For this review, take the finished solid that the model builds, in its own axes (mm). A direction names the side the tool comes from. Give positions to 0.01 mm unless a question says otherwise; leave off trailing zeros. Write each loop counter-clockwise with the first axis right and the second up, starting at its lowest first coordinate (ties: lowest second). Pieces come first, ordered by that corner, then holes. Notation, with made-up numbers: M 7.5,89.5 L 59.5,89.5 A14 cw 59.5,116.5 Z; hole C 72,-34 d1. An arc over 180 degrees is marked long. One line per item, written item: value. Start each with the question number.
Item 1: Consider section C-C, the plane y = -7.5. Write out the cut boundary in (x, z), and give its area (3 significant figures).
Item 2: Consider section A-A, the plane z = 0. Write out the cut boundary in (x, y).
Item 3: Consider section B-B, the plane x = 0. Write out the cut boundary in (y, z).
Item 4: Mouldability with a two-part tool opening along Y and no side actions: class faces 1 (the face through (4, 0, 7)), 2 (the face through (4, -20, 7)), 3 (the face through (-6.347, -5.746, 5.319)) as released by +Y, released by -Y, zero draft, split by the parting line, or undercut.
Item 5: Clearance check with flat-ended pins moving along their axes: pin 1 Ø1 at (y, z) = (-3, 6.5) entering from -X; pin 2 Ø6 at (x, y) = (0, -7.5) entering from +Z; pin 3 Ø4 at (y, z) = (-3.5, 7) entering from -X; pin 4 Ø2 at (y, z) = (-4.5, -5.5) entering from +X. State where each tip first meets the part, or that it passes through.
Item 6: To check wall thickness, follow probe 1 along Y at (x, z) = (0, 8.1); probe 2 along X at (y, z) = (-3.5, 0.25). State the ranges of each line that lie inside material, in increasing order.
Item 7: Tool access review of faces 4 (the face through (-1.8, -6.9, 8.2)), 5 (the face through (4.153, -9.86, -7.985)): name each direction out of +Z, -Z, +X, -X, +Y, -Y from which nothing blocks a thin tool from reaching the whole face with its end or side.
Item 8: Consider section D-D, the plane y = -12.5. Write out the cut boundary in (x, z), and give its area (3 significant figures).
```python
from build123d import *

# Parameters (mm, degrees)
F0_R     = 9
F0_R_2   = 7.75
F1_DEPTH = 20
F4_D     = 3.7973
F4_DEPTH = 3.021
F4_START = 0.20255
F4_TIP   = 1.1408240143
F8_D     = 3.7973
F8_DEPTH = 2
F8_START = 0.20255
F8_TIP   = 1.1408240143


with BuildPart() as f1:
    # F0 (on Front) → F1 (new body)
    with BuildSketch(Plane.XZ):
        Circle(F0_R)
        Circle(F0_R_2, mode=Mode.SUBTRACT)
    extrude(amount=F1_DEPTH)

    # F4
    # its depths count from where the whole tool has entered the part; down to there all is cleared
    with Locations(Plane.XY.offset(9).offset(-F4_START)):
        with Locations((0, -7.5)):
            Hole(F4_D / 2, depth=F4_DEPTH)
            with Locations((0, 0, -(F4_DEPTH + F4_TIP / 2))):  # 118° drill point
                Cone(0, F4_D / 2, F4_TIP, mode=Mode.SUBTRACT)

    # F8
    # its depths count from where the whole tool has entered the part; down to there all is cleared
    with Locations(Plane(origin=(-6.3639610307, 0, 6.3639610307), x_dir=(0, -1, 0), z_dir=(-0.7071067812, 0, 0.7071067812)).offset(-F8_START)):
        with Locations((7.5, 0)):
            Hole(F8_D / 2, depth=F8_DEPTH)
            with Locations((0, 0, -(F8_DEPTH + F8_TIP / 2))):  # 118° drill point
                Cone(0, F8_D / 2, F8_TIP, mode=Mode.SUBTRACT)


solid = f1.part
```
Model answer:
1. outline: M -7.56,4.88 A9 ccw long 1.9,8.8 L 1.9,7.51 A7.75 cw long -6.66,3.97 Z; M -4.88,7.56 L -3.97,6.66 A7.75 cw -1.9,7.51 L -1.9,8.8 A9 ccw Z
1. area: 56.2 mm2
2. outline: M -9,-20 L -7.75,-20 L -7.75,0 L -9,0 Z; M 7.75,-20 L 9,-20 L 9,0 L 7.75,0 Z
3. outline: M -20,-9 L 0,-9 L 0,-7.75 L -20,-7.75 Z; M -20,7.75 L -9.4,7.75 L -9.4,9 L -20,9 Z; M -5.6,7.75 L 0,7.75 L 0,9 L -5.6,9 Z
4. face 1: released by +Y
4. face 2: released by -Y
4. face 3: undercut
5. pin 1: stops at x = -6.71
5. pin 2: stops at z = 9
5. pin 3: stops at x = -7.48
5. pin 4: stops at x = 7.79
6. probe 1: y = -20 to -9.4, -5.6 to 0
6. probe 2: x = -9 to -7.75, 7.75 to 9
7. face 4: +Z
7. face 5: +Y, -Y
8. outline: C 0,0 d18; hole C 0,0 d15.5
8. area: 65.8 mm2
